The figure shows three views and two pictorial views of one solid part (mm, origin at its lowest corner). Answer the questions. A direction names the side the tool comes from. Give positions to 0.01 mm unless a question says otherwise; leave off trailing zeros. Order: outer loops, then holes, each group sorted by start corner. A loop starts at its lowest first (then second) coordinate and runs counter-clockwise, first axis right, second up. Notation, with made-up numbers: (17.5, -17.5) - (72.5, -17.5) arc R33 cw to (72.5, 21.5) - close; hole circle Ø5 at (86.5, 72.25). An arc over 180 degrees is marked (long way). Answer as a JSON object with one key per item and string values. Group by question number.
Q1. Consider line 1 (Y direction, x = 22.5, z = 4); line 2 (X direction, y = 21, z = 8.75); line 3 (Y direction, x = 22.5, z = 8.4). Determine where each line is inside the solid, lowest interval first.
Q2. The mould has two halves that part along X. Classify the marked faces 1, 2 and 3: released by +X, released by -X, zero draft, split by the parting line, or undercut.
Q3. Given pin 1 (6.5 mm diameter, centred on x = 9.5, y = 22.5, fed in from -Z); pin 2 (3 mm diameter, centred on x = 35, y = 22.5, fed in from +Z); pin 3 (6 mm diameter, centred on y = 7, z = 2, fed in from -X); pin 4 (1.5 mm diameter, centred on x = 27, z = 6.5, fed in from +Y), each flat-ended and moving along its own axis, determine where each tip first touches the part or whether it passes through.
Q4. A cutting plane is placed at B-B, the plane z = 2.25. Give the vertices of the cut face in (x, y).
Q5. A cutting plane is placed at A-A, the plane y = 22.5. Give the vertices of the cut face in (x, z).
Q6. For the marked faces 4 and 5, determine the directions among +Z, -Z, +X, -X, +Y, -Y from which every point of the face is accessible in a straight line to the end or side of a thin tool.
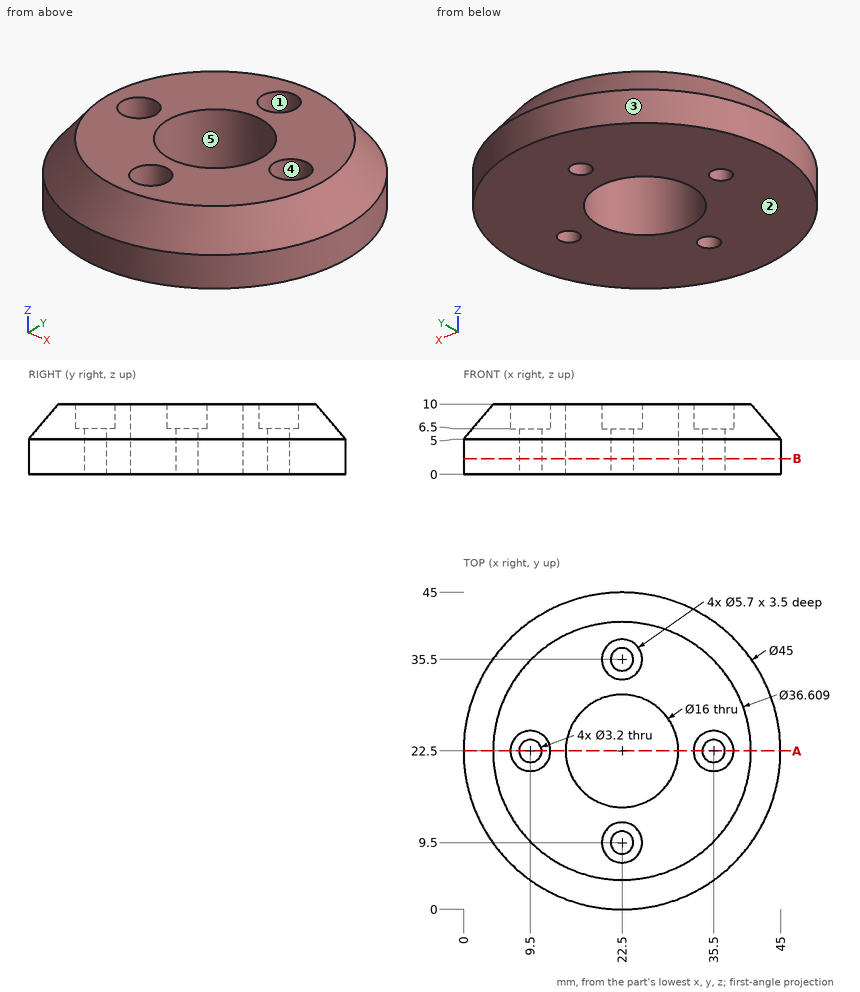
Reply:
{
 "1": {"line 1": "y = 0 to 7.9, 11.1 to 14.5, 30.5 to 33.9, 37.1 to 45", "line 2": "x = 3.2 to 7.08, 11.92 to 14.64, 30.36 to 33.08, 37.92 to 41.8", "line 3": "y = 2.85 to 6.65, 12.35 to 14.5, 30.5 to 32.65, 38.35 to 42.15"},
 "2": {"face 1": "undercut", "face 2": "zero draft", "face 3": "split by the parting line"},
 "3": {"pin 1": "stops at z = 0", "pin 2": "stops at z = 6.5", "pin 3": "stops at x = 3.79", "pin 4": "stops at y = 43.92"},
 "4": {"outline": "circle Ø45 at (22.5, 22.5); hole circle Ø3.2 at (9.5, 22.5); hole circle Ø16 at (22.5, 22.5); hole circle Ø3.2 at (22.5, 9.5); hole circle Ø3.2 at (22.5, 35.5); hole circle Ø3.2 at (35.5, 22.5)"},
 "5": {"outline": "(0, 0) - (7.9, 0) - (7.9, 6.5) - (6.65, 6.5) - (6.65, 10) - (4.2, 10) - (0, 5) - close; (11.1, 0) - (14.5, 0) - (14.5, 10) - (12.35, 10) - (12.35, 6.5) - (11.1, 6.5) - close; (30.5, 0) - (33.9, 0) - (33.9, 6.5) - (32.65, 6.5) - (32.65, 10) - (30.5, 10) - close; (37.1, 0) - (45, 0) - (45, 5) - (40.8, 10) - (38.35, 10) - (38.35, 6.5) - (37.1, 6.5) - close"},
 "6": {"face 4": "+Z", "face 5": "+Z, -Z"}
}
